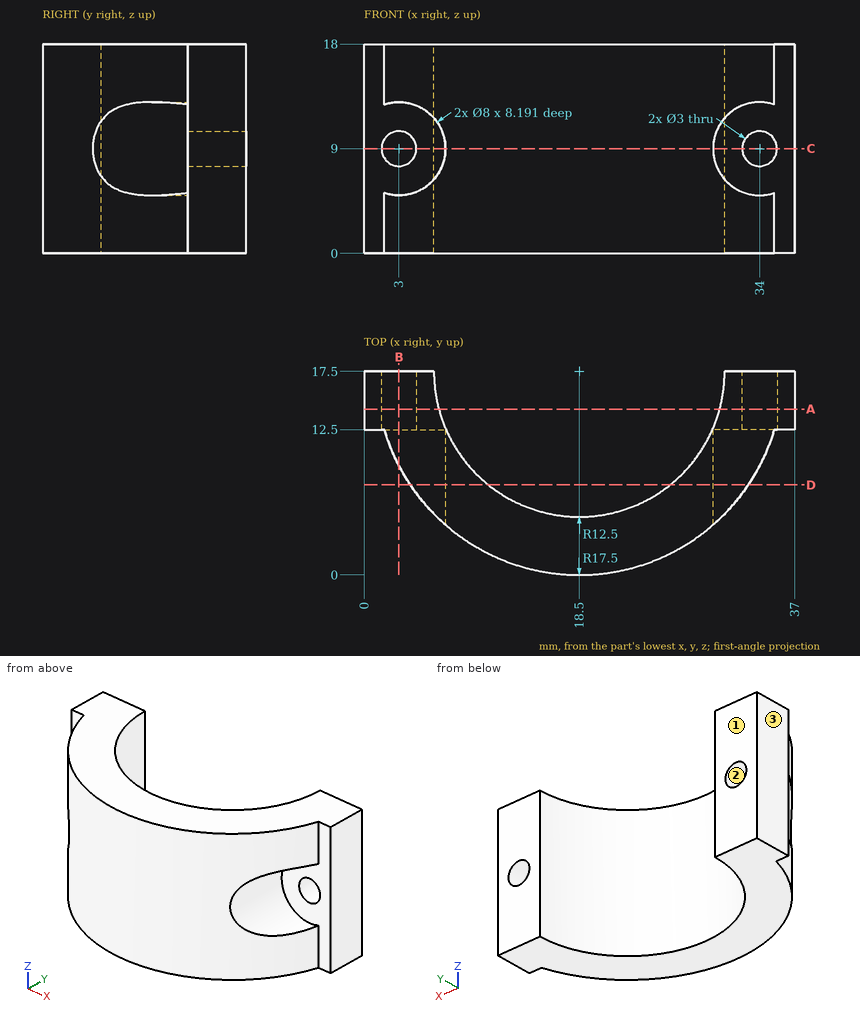
The figure shows three views and two pictorial views of one solid part (mm, origin at its lowest corner). Answer the questions. Round coordinates to 2 decimals unless told otherwise and drop trailing zeros. Write each loop counter-clockwise with the first axis right and the second up, starting at its lowest first coordinate (ties: lowest second). Pieces come first, ordered by that corner, then holes. Notation, with made-up numbers: M -29,61 L 19,61 A5 ccw 19,66 Z; hole C -1.75,37.25 d5. An arc over 180 degrees is marked long. Use a Markdown table: item, result.
1) Straight lines are drawn through the part: line 1 along Z through (x, y) = (34, 16.2); line 2 along X through (y, z) = (16, 8); line 3 along X through (y, z) = (16, 9.25). For each, find the intervals that lie inside material, in ascending order. Write a range as [from, to].
Answers follow:
| item | result |
|---|---|
| line 1 | z = [0, 7.5], [10.5, 18] |
| line 2 | x = [0, 1.88], [4.12, 6.09], [30.91, 32.88], [35.12, 37] |
| line 3 | x = [0, 1.52], [4.48, 6.09], [30.91, 32.52], [35.48, 37] |
2) For a pull along X with two mould halves and no side action, classify the marked faces 1, 2 and 3 as pulls with the +X half, pulls with the -X half, needs draft (parallel to the pull), parting line crosses it, or undercut.
Answers follow:
| item | result |
|---|---|
| face 1 | needs draft |
| face 2 | undercut |
| face 3 | pulls with the -X half |
3) Flat-ended cylindrical pins translate along their axes: pin 1 (4 mm diameter, centred on y = 8, z = 12.5, fed in from +X); pin 2 (7 mm diameter, centred on x = 3, z = 9, fed in from -Y); pin 3 (3 mm diameter, centred on y = 2.5, z = 8, fed in from +X). Find the tip coordinate at first contact, or state that the pin passes through.
Answers follow:
| item | result |
|---|---|
| pin 1 | stops at x = 34.28 |
| pin 2 | stops at y = 12.5 |
| pin 3 | stops at x = 29.64 |
4) The part is cut by section B-B (x = 3). Write down the section's boundary in (y, z), plus the area to 3 significant figures.
Answers follow:
| item | result |
|---|---|
| outline | M 9.38,0 L 17.5,0 L 17.5,7.5 L 12.5,7.5 L 12.5,5 L 9.38,5 Z; M 9.38,13 L 12.5,13 L 12.5,10.5 L 17.5,10.5 L 17.5,18 L 9.38,18 Z |
| area | 106 mm2 |
5) The part is cut by section D-D (y = 7.75). Write down the section's boundary in (x, z), plus the area to 3 significant figures.
Answers follow:
| item | result |
|---|---|
| outline | M 3.97,0 L 10.68,0 L 10.68,18 L 3.97,18 L 3.97,12.88 A4 cw 3.97,5.12 Z; M 26.32,0 L 33.03,0 L 33.03,5.12 A4 cw 33.03,12.88 L 33.03,18 L 26.32,18 Z |
| area | 207 mm2 |
6) The part is cut by section A-A (y = 14.25). Write down the section's boundary in (x, z), plus the area to 3 significant figures.
Answers follow:
| item | result |
|---|---|
| outline | M 0,0 L 6.43,0 L 6.43,18 L 0,18 Z; M 30.57,0 L 37,0 L 37,18 L 30.57,18 Z; hole C 3,9 d3; hole C 34,9 d3 |
| area | 217 mm2 |
7) The part is cut by section C-C (z = 9). Write down the section's boundary in (x, y).
Answers follow:
| item | result |
|---|---|
| outline | M 0,12.5 L 1.5,12.5 L 1.5,17.5 L 0,17.5 Z; M 4.5,12.5 L 7,12.5 L 7,4.31 A17.5 ccw 30,4.31 L 30,12.5 L 32.5,12.5 L 32.5,17.5 L 31,17.5 A12.5 cw 6,17.5 L 4.5,17.5 Z; M 35.5,12.5 L 37,12.5 L 37,17.5 L 35.5,17.5 Z |
